from build123d import *

# Parameters (mm, degrees)
HEAD_CUT_DEPTH      = 4.1750001
HEAD_CUT_DEPTH_BACK = 4.1750001
SKETCH6_R           = 1.778
HOLE_CUT_DEPTH      = 3.0828001
HOLE_CUT_DEPTH_BACK = 3.0828001


with BuildPart() as part:
    # Sketch3 → Body Revolve (revolve)
    with BuildSketch(Plane(origin=(0, 0, 0), x_dir=(0, 0, -1), z_dir=(1, 0, 0))):
        with BuildLine():
            Line((19.05, 0), (19.05, 1.685925))
            Line((19.05, 1.685925), (18.653125, 2.0828))
            Line((18.653125, 2.0828), (5.55625, 2.0828))
            ThreePointArc((5.55625, 2.0828), (4.060634728, 2.894312369), (2.382352325, 3.175))
            Line((2.382352325, 3.175), (-2.38125, 3.175))
            Line((-2.38125, 3.175), (-4.477145765, 2.961701818))
            ThreePointArc((-4.477145765, 2.961701818), (-4.680597677, 2.858671264), (-4.7625, 2.645833333))
            Line((-4.7625, 2.645833333), (-4.7625, 0))
            Line((-4.7625, 0), (19.05, 0))
        make_face()
    revolve(axis=Axis((0, 0, 4.7625), (0, 0, -1)))

    # Sketch5 → Head Cut (cut, two sides)
    with BuildSketch(Plane(origin=(0, 0, 0), x_dir=(1, 0, 0), z_dir=(0, 1, 0))) as head_cut_sk:
        with BuildLine():
            Line((-3.9624, 5.55625), (-3.9624, -4.7625))
            Line((-3.9624, -4.7625), (-0.7874, -4.7625))
            Line((-0.7874, -4.7625), (-0.7874, 2.382352325))
            ThreePointArc((-0.7874, 2.382352325), (-1.12371822, 4.096389053), (-2.0828, 5.55625))
            Line((-2.0828, 5.55625), (-3.9624, 5.55625))
        make_face()
        with BuildLine():
            Line((2.0828, 5.55625), (3.9624, 5.55625))
            Line((3.9624, 5.55625), (3.9624, -4.7625))
            Line((3.9624, -4.7625), (0.7874, -4.7625))
            Line((0.7874, -4.7625), (0.7874, 2.382352325))
            ThreePointArc((0.7874, 2.382352325), (1.12371822, 4.096389053), (2.0828, 5.55625))
        make_face()
    extrude(amount=HEAD_CUT_DEPTH, mode=Mode.SUBTRACT)
    extrude(head_cut_sk.sketch, amount=-HEAD_CUT_DEPTH_BACK, mode=Mode.SUBTRACT)

    # Sketch6 → Hole Cut (cut, two sides)
    with BuildSketch(Plane(origin=(0, 0, 0), x_dir=(0, 0, -1), z_dir=(1, 0, 0))) as hole_cut_sk:
        Circle(SKETCH6_R)
    extrude(amount=HOLE_CUT_DEPTH, mode=Mode.SUBTRACT)
    extrude(hole_cut_sk.sketch, amount=-HOLE_CUT_DEPTH_BACK, mode=Mode.SUBTRACT)


solid = part.part
Verification items for the finished model (mm, model axes). A direction names the side the tool comes from. Round coordinates to 2 decimals unless told otherwise and drop trailing zeros. Write each loop counter-clockwise with the first axis right and the second up, starting at its lowest first coordinate (ties: lowest second). Pieces come first, ordered by that corner, then holes.
(1) Mould release check, pull along Y, two halves, no side actions. Record for faces 4 (the cylindrical face through (-0.985, -0.043, -3.705)), 5 (the conical face through (-0.012, 3.067, 3.444)), 6 (the cylindrical face through (0.011, -1.736, 0.385)), 7 (the cylindrical face through (0.626, 1.987, -12.013)): pulls with the +Y half, pulls with the -Y half, needs draft (parallel to the pull), parting line crosses it, or undercut.
Returned:
face 4: needs draft
face 5: pulls with the +Y half
face 6: undercut
face 7: parting line crosses it
(2) Depth check by flat-ended pin: pin 1 Ø2 at (y, z) = (-2, -1) entering from -X; pin 2 Ø1.8 at (y, z) = (1, 3) entering from +X. Enter the tip coordinate at first touch or a pass-through.
Returned:
pin 1: stops at x = -0.79
pin 2: stops at x = 0.79
(3) Material ranges on line 1 (Z direction, x = 0.3, y = 0); line 2 (Y direction, x = -0.25, z = 0); line 3 (X direction, y = 1, z = 3.25), recorded low to high.
Returned:
line 1: z = -19.05 to -1.78, 1.78 to 4.76
line 2: y = -3.17 to -1.78, 1.78 to 3.17
line 3: x = -0.79 to 0.79
(4) Section check B-B (z = -13.75). Enter the section's corners in (x, y), plus the area to 3 significant figures.
Returned:
outline: circle Ø4.17 at (0, 0)
area: 13.6 mm2
(5) Section check A-A (z = 0). Enter the section's corners in (x, y) (3 decimals), plus the area to 3 significant figures.
Returned:
outline: (-0.787, -3.076) arc R3.175 ccw to (0.787, -3.076) - (0.787, -1.778) - (-0.787, -1.778) - close; (-0.787, 1.778) - (0.787, 1.778) - (0.787, 3.076) arc R3.175 ccw to (-0.787, 3.076) - close
area: 4.30 mm2
(6) Access from +Z, -Z, +X, -X, +Y, -Y to the whole of each face (thin tool, end or side, straight path). Record for faces 1 (the flat face through (0, 0, -19.05)), 2 (the flat face through (-0.787, 0, 2)), 3 (the flat face through (0.787, 0, 2)).
Returned:
face 1: -Z, +X, -X, +Y, -Y
face 2: +Z, -X, +Y, -Y
face 3: +Z, +X, +Y, -Y
